Could you check a few things on this model? Use its own coordinates, in mm. A direction names the side the tool comes from. Coordinates: 2 decimals unless noted, no trailing zeros. Order: outer loops, then holes, each group sorted by start corner. A loop starts at its lowest first (then second) coordinate and runs counter-clockwise, first axis right, second up. Notation, with made-up numbers: (57, 2) - (97, 2) arc R19 cw to (97, 32) - close; hole circle Ø3 at (52.5, 79). An arc over 180 degrees is marked (long way). One line per item, written item: value. Start each with the question number.
from build123d import *

# Parameters (mm, degrees)
F1_DEPTH = 3.3


with BuildPart() as f1:
    # F0 (on Top) → F1 (new body)
    with BuildSketch(Plane.XY):
        with BuildLine():
            ThreePointArc((2, 3.4641016151), (3.4641016151, 2), (4, 0))
            Line((4, 0), (4.85, 0))
            ThreePointArc((4.85, 0), (4.2002232084, 2.425), (2.425, 4.2002232084))
            Line((2.425, 4.2002232084), (2, 3.4641016151))
        make_face()
        with BuildLine():
            ThreePointArc((1.9625, 3.3991497099), (3.3991497099, 1.9625), (3.925, 0))
            Line((3.925, 0), (4, 0))
            ThreePointArc((4, 0), (3.4641016151, 2), (2, 3.4641016151))
            Line((2, 3.4641016151), (1.9625, 3.3991497099))
        make_face()
        with BuildLine():
            ThreePointArc((-1.9625, 3.3991497099), (0, 3.925), (1.9625, 3.3991497099))
            Line((1.9625, 3.3991497099), (2, 3.4641016151))
            ThreePointArc((2, 3.4641016151), (0, 4), (-2, 3.4641016151))
            Line((-2, 3.4641016151), (-1.9625, 3.3991497099))
        make_face()
        with BuildLine():
            ThreePointArc((-3.925, 0), (-3.3991497099, 1.9625), (-1.9625, 3.3991497099))
            Line((-1.9625, 3.3991497099), (-2, 3.4641016151))
            ThreePointArc((-2, 3.4641016151), (-3.4641016151, 2), (-4, 0))
            Line((-4, 0), (-3.925, 0))
        make_face()
        with BuildLine():
            ThreePointArc((-4, 0), (-3.4641016151, 2), (-2, 3.4641016151))
            Line((-2, 3.4641016151), (-2.425, 4.2002232084))
            ThreePointArc((-2.425, 4.2002232084), (-4.2002232084, 2.425), (-4.85, 0))
            Line((-4.85, 0), (-4, 0))
        make_face()
        with BuildLine():
            Line((-2, -3.4641016151), (-1.9625, -3.3991497099))
            ThreePointArc((-1.9625, -3.3991497099), (-3.3991497099, -1.9625), (-3.925, 0))
            Line((-3.925, 0), (-4, 0))
            ThreePointArc((-4, 0), (-3.4641016151, -2), (-2, -3.4641016151))
        make_face()
        with BuildLine():
            Line((2.425, -4.2002232084), (2, -3.4641016151))
            ThreePointArc((2, -3.4641016151), (0, -4), (-2, -3.4641016151))
            Line((-2, -3.4641016151), (-2.425, -4.2002232084))
            ThreePointArc((-2.425, -4.2002232084), (0, -4.85), (2.425, -4.2002232084))
        make_face()
        with BuildLine():
            Line((2, -3.4641016151), (1.9625, -3.3991497099))
            ThreePointArc((1.9625, -3.3991497099), (0, -3.925), (-1.9625, -3.3991497099))
            Line((-1.9625, -3.3991497099), (-2, -3.4641016151))
            ThreePointArc((-2, -3.4641016151), (0, -4), (2, -3.4641016151))
        make_face()
        with BuildLine():
            Line((4, 0), (3.925, 0))
            ThreePointArc((3.925, 0), (3.3991497099, -1.9625), (1.9625, -3.3991497099))
            Line((1.9625, -3.3991497099), (2, -3.4641016151))
            ThreePointArc((2, -3.4641016151), (3.4641016151, -2), (4, 0))
        make_face()
    extrude(amount=F1_DEPTH)


solid = f1.part
Q1. I want a section at B-B on x = -1.75. Please give me the cut outline in (y, z), then the cut area to 3 significant figures.
Q2. I want a section at A-A on y = 2. Please give me the cut outline in (x, z).
Q3. I'm going to push flat-ended pins straight in: pin 1 (1 mm diameter, centred on x = -2.5, z = 0.5, fed in from -Y); pin 2 (0.7 mm diameter, centred on x = 4.5, z = 1.5, fed in from -Y). Where does each tip first touch, or does it pass through?
Q4. If I drill on L1, parallel to Y at x = -3.5, z = 2.1; L2, parallel to X at y = 0.25, z = 0.2; L3, parallel to X at y = 2.25, z = 1.65, over which ranges is the centre line in solid material (lowest first)?
Q5. Which directions (+Z, -Z, +X, -X, +Y, -Y) give clear straight access to the entire face, cutting with the end or side of a thin tool? Please do faces 1 (the cylindrical face through (-0.04, -4.85, 1.63)), 2 (the flat face through (4.4, 0, 1.6)), 3 (the flat face through (-4.4, 0, 1.6)).
Values follow:
1. outline: (-4.52, 0) - (-3.51, 0) - (-3.51, 3.3) - (-4.52, 3.3) - close; (3.51, 0) - (3.6, 0) - (3.6, 3.3) - (3.51, 3.3) - close
1. area: 3.61 mm^2
2. outline: (-4.42, 0) - (-3.38, 0) - (-3.38, 3.3) - (-4.42, 3.3) - close; (3.38, 0) - (4.42, 0) - (4.42, 3.3) - (3.38, 3.3) - close
3. pin 1: stops at y = -4.42
3. pin 2: stops at y = 0
4. L1: y = -1.94 to -1.78, 1.78 to 3.36
4. L2: x = -4.84 to -3.92, 3.92 to 4.84
4. L3: x = -4.3 to -3.22, 3.22 to 4.3
5. face 1: +Z, -Z, -Y
5. face 2: +Z, -Z, +X, -Y
5. face 3: +Z, -Z, -X, -Y
